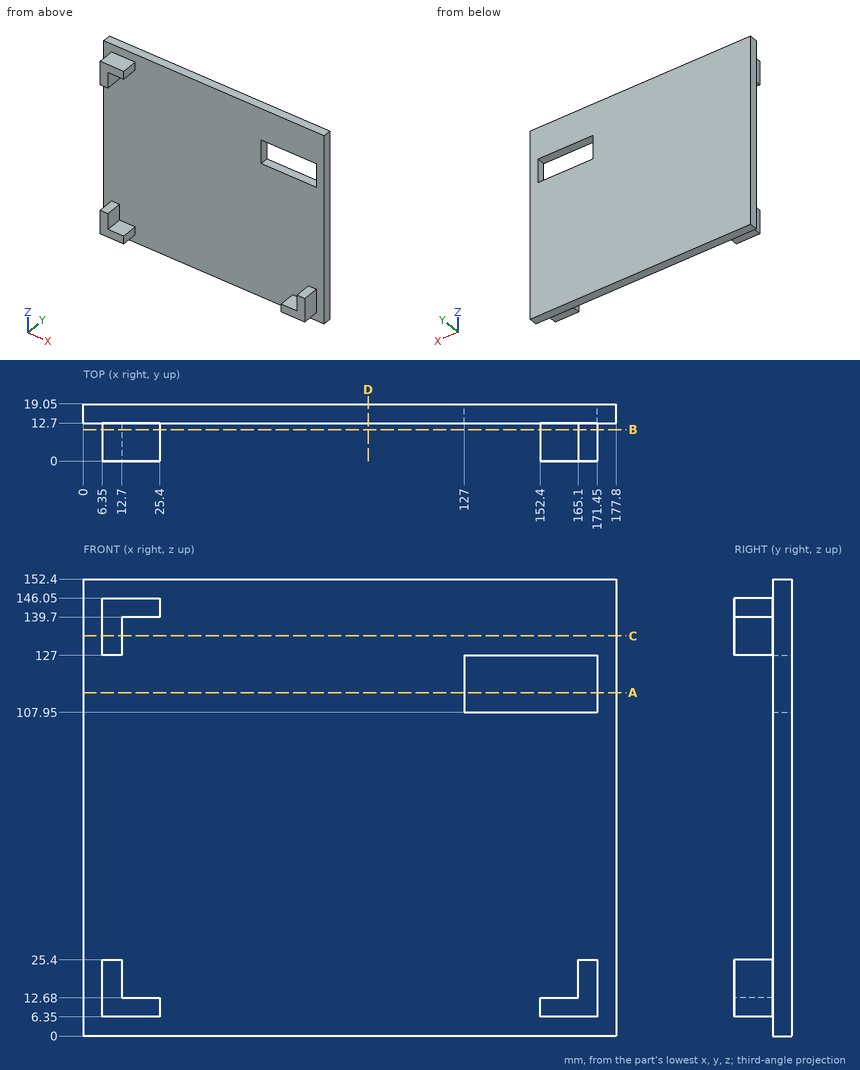
Study the drawing (mm; zero at the part's minimum x, y, z) and answer. Give positions to 0.01 mm unless a question says otherwise; leave off trailing zeros. Write each loop counter-clockwise with the first axis right and the second up, starting at its lowest first coordinate (ties: lowest second). Pieces come first, ordered by that corner, then holes. Notation, with made-up numbers: (24, -37.5) -> (76, -37.5) arc R19 cw to (76, -8.5) -> close; hole circle Ø10 at (79, 17). An arc over 180 degrees is marked (long way). Answer as a JSON object with one key per item and string values. Group by question number.
1) Find section D-D (x = 95). Write down the section's boundary in (y, z), and give its area (3 significant figures).
2) Consider L1, parallel to Z at x = 148.5, y = 16.75; L2, parallel to Y at x = 160, z = 128; L3, parallel to X at y = 6.75, z = 129.5. Determine where each line is inside the solid, lowest interval first. Write a range as from..to.
3) Find section C-C (z = 133.5). Write down the section's boundary in (x, y).
4) Find section A-A (z = 114.5). Write down the section's boundary in (x, y), and give its area (3 significant figures).
5) Each of these flat-tipped pins is pushed along its axis until it touches: P1, Ø10, axis at y = 6.5, z = 21, coming from the -X side; P2, Ø7, axis at x = 9, y = 6, coming from the -Z side; P3, Ø10, axis at y = 7.5, z = 18.5, coming from the +X side. Where does it stop, or does it pass through?
6) Find section B-B (y = 10.5). Write down the section's boundary in (x, z), and give its area (3 significant figures).
Values follow:
{
 "1": {"outline": "(12.7, 0) -> (19.05, 0) -> (19.05, 152.4) -> (12.7, 152.4) -> close", "area": "968 mm2"},
 "2": {"L1": "z = 0..107.95, 127..152.4", "L2": "y = 12.7..19.05", "L3": "x = 6.35..12.7"},
 "3": {"outline": "(0, 12.7) -> (6.35, 12.7) -> (6.35, 0) -> (12.7, 0) -> (12.7, 12.7) -> (177.8, 12.7) -> (177.8, 19.05) -> (0, 19.05) -> close"},
 "4": {"outline": "(0, 12.7) -> (127, 12.7) -> (127, 19.05) -> (0, 19.05) -> close; (171.45, 12.7) -> (177.8, 12.7) -> (177.8, 19.05) -> (171.45, 19.05) -> close", "area": "847 mm2"},
 "5": {"P1": "stops at x = 6.35", "P2": "stops at z = 6.35", "P3": "stops at x = 171.45"},
 "6": {"outline": "(6.35, 6.35) -> (25.4, 6.35) -> (25.4, 12.68) -> (12.7, 12.68) -> (12.7, 25.4) -> (6.35, 25.4) -> close; (6.35, 127) -> (12.7, 127) -> (12.7, 139.7) -> (25.4, 139.7) -> (25.4, 146.05) -> (6.35, 146.05) -> close; (152.4, 6.35) -> (171.45, 6.35) -> (171.45, 25.4) -> (165.1, 25.4) -> (165.1, 12.68) -> (152.4, 12.68) -> close", "area": "604 mm2"}
}
